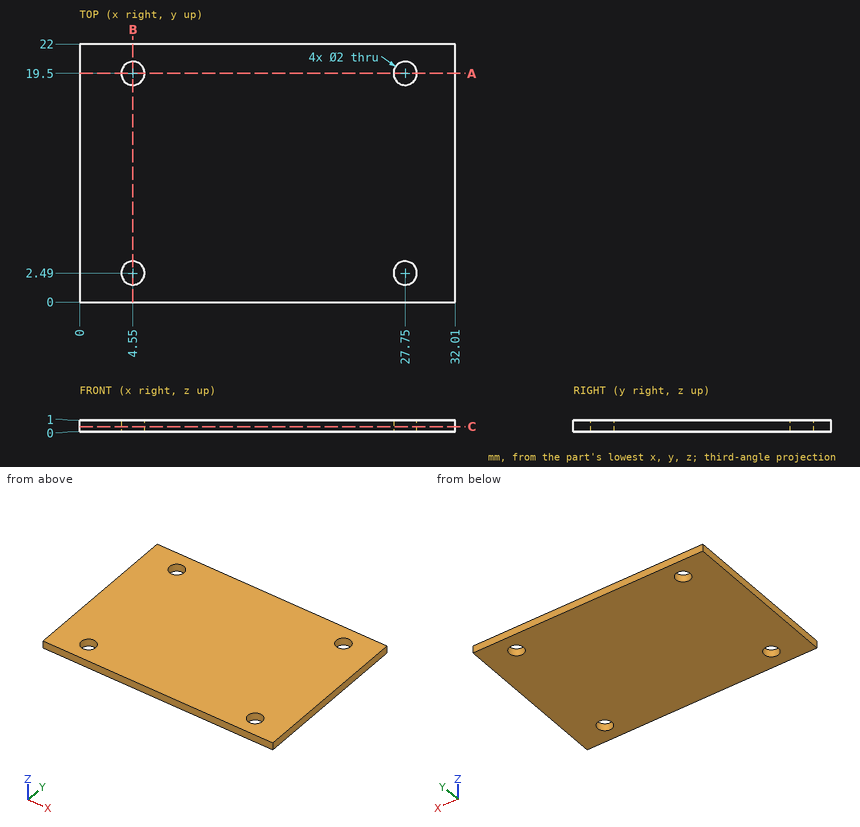
The drawing under review shows one solid part. Ordinate dimensions are in mm from its lowest x, y, z. Give positions to 0.01 mm unless a question says otherwise; leave off trailing zeros. Loops run counter-clockwise (first coordinate to the right, second up) from the corner with the lowest first, then second, coordinate; pieces in that order, holes last. Notation, with made-up numbers: M 24,-10 L 67,-10 A31 cw 67,16 Z; hole C 50.5,-32.75 d10. An arc over 180 degrees is marked long. One line per item, written item: value. Start each with the question number.
Q1. For L1, parallel to X at y = 19.5, z = 0.7; L2, parallel to Y at x = 27.75, z = 0.2; L3, parallel to X at y = 2, z = 0.9, list the stretches that pass through material, from the lowest coordinate up.
Q2. Add section C-C (z = 0.45). Give the boundary of the cut face in (x, y), and give its area (3 significant figures).
Q3. Add section A-A (y = 19.5). Give the boundary of the cut face in (x, z).
Q4. Add section B-B (x = 4.55). Give the boundary of the cut face in (y, z), and give its area (3 significant figures).
Reply:
1. L1: 0 to 3.55, 5.55 to 26.75, 28.75 to 32.01
1. L2: 0 to 1.49, 3.49 to 18.5, 20.5 to 22
1. L3: 0 to 3.68, 5.42 to 26.88, 28.62 to 32.01
2. outline: M 0,0 L 32.01,0 L 32.01,22 L 0,22 Z; hole C 4.55,2.49 d2; hole C 4.55,19.5 d2; hole C 27.75,2.49 d2; hole C 27.75,19.5 d2
2. area: 692 mm²
3. outline: M 0,0 L 3.55,0 L 3.55,1 L 0,1 Z; M 5.55,0 L 26.75,0 L 26.75,1 L 5.55,1 Z; M 28.75,0 L 32.01,0 L 32.01,1 L 28.75,1 Z
4. outline: M 0,0 L 1.49,0 L 1.49,1 L 0,1 Z; M 3.49,0 L 18.5,0 L 18.5,1 L 3.49,1 Z; M 20.5,0 L 22,0 L 22,1 L 20.5,1 Z
4. area: 18.0 mm²
